Can you work these out from the model? Positions are in its coordinate system, mm. A direction names the side the tool comes from. Give positions to 0.01 mm unless a question says otherwise; leave off trailing zeros. Write each loop counter-clockwise with the first axis right and the second up, starting at its lowest first coordinate (ties: lowest second). Pieces come first, ordered by that corner, then holes.
```python
from build123d import *

# Parameters (mm, degrees)
BOSS_EXTRUDE1_DEPTH = 100
CUT_EXTRUDE1_DEPTH  = 100
BOSS_EXTRUDE2_DEPTH = 15
SKETCH4_W           = 40
SKETCH4_H           = 35
CUT_EXTRUDE2_DEPTH  = 137.950721064
SKETCH5_W           = 20
SKETCH5_H           = 15
BOSS_EXTRUDE3_DEPTH = 10
SKETCH6_W           = 20
SKETCH6_H           = 15
BOSS_EXTRUDE4_DEPTH = 10


with BuildPart() as part:
    # Sketch1 → Boss-Extrude1 (new body)
    with BuildSketch(Plane(origin=(0, 0, 0), x_dir=(1, 0, 0), z_dir=(0, 1, 0))):
        with BuildLine():
            Line((-10, 54.591666031), (-10, 39.591666031))
            Line((-10, 39.591666031), (-5, 39.591666031))
            Line((-5, 39.591666031), (-5, 24.591666031))
            Line((-5, 24.591666031), (-10, 24.591666031))
            Line((-10, 24.591666031), (-10, 0))
            ThreePointArc((-10, 0), (-7.071067812, -7.071067812), (0, -10))
            Line((0, -10), (20, -10))
            Line((20, -10), (20, -25))
            Line((20, -25), (-20, -25))
            Line((-20, -25), (-20, -51.771130952))
            ThreePointArc((-20, -51.771130952), (-55.256322222, 5.195079839), (-10, 54.591666031))
        make_face()
    extrude(amount=BOSS_EXTRUDE1_DEPTH)

    # Sketch2 → Cut-Extrude1 (cut)
    with BuildSketch(Plane(origin=(0, 0, 10), x_dir=(-1, 0, 0), z_dir=(0, 0, -1))):
        with BuildLine():
            Line((-5, 90.003555636), (-5, 10.003555636))
            ThreePointArc((-5, 10.003555636), (-10, 5.003555636), (-15, 10.003555636))
            Line((-15, 10.003555636), (-15, 90.003555636))
            ThreePointArc((-15, 90.003555636), (-10, 95.003555636), (-5, 90.003555636))
        make_face()
    extrude(amount=-CUT_EXTRUDE1_DEPTH, mode=Mode.SUBTRACT)

    # Sketch3 → Boss-Extrude2 (add)
    with BuildSketch(Plane(origin=(0, 100, 0), x_dir=(1, 0, 0), z_dir=(0, 1, 0))):
        with BuildLine():
            Line((20, -25), (20, -20))
            Line((20, -20), (-55.356937984, -3.982388364))
            ThreePointArc((-55.356937984, -3.982388364), (-44.616230288, -33.009725763), (-20, -51.771130952))
            Line((-20, -51.771130952), (-20, -25))
            Line((-20, -25), (20, -25))
        make_face()
    extrude(amount=BOSS_EXTRUDE2_DEPTH)

    # Sketch4 → Cut-Extrude2 (cut, through all)
    with BuildSketch(Plane(origin=(-5, 0, 0), x_dir=(0, 0, -1), z_dir=(1, 0, 0))):
        with Locations((34.591666031, 52.5)):
            Rectangle(SKETCH4_W, SKETCH4_H)
    extrude(amount=-CUT_EXTRUDE2_DEPTH, mode=Mode.SUBTRACT)

    # Sketch5 → Boss-Extrude3 (add)
    with BuildSketch(Plane(origin=(0, 100, 0), x_dir=(1, 0, 0), z_dir=(0, 1, 0))):
        with Locations((-15, 32.091666031)):
            Rectangle(SKETCH5_W, SKETCH5_H)
    extrude(amount=BOSS_EXTRUDE3_DEPTH)

    # Sketch6 → Boss-Extrude4 (add)
    with BuildSketch(Plane.XZ):
        with Locations((-15, -32.091666031)):
            Rectangle(SKETCH6_W, SKETCH6_H)
    extrude(amount=BOSS_EXTRUDE4_DEPTH)


solid = part.part
```
1) For faces 1 (the face through (0, 57, 25)), 2 (the face through (-8, 99, -24.592)), 3 (the face through (-24, 70, -30)), 4 (the face through (-5, 90, -32)), 5 (the face through (9.89, 5.005, 17.395)), which set-ups out of +Z, -Z, +X, -X, +Y, -Y let a thin tool reach every point of the face, with its end or its side?
Values follow:
face 1: +Z, +X, +Y, -Y
face 2: +X, +Y
face 3: -Z, +X, -X
face 4: -Z, +X, +Y, -Y
face 5: +Z, -Z
2) Suppose I cut it at C-C on x = 8. Write out the boundary of the cut face in (y, z).
Values follow:
outline: (0, 10) - (5.42, 10) - (5.42, 25) - (0, 25) - close; (94.59, 10) - (100, 10) - (100, 17.45) - (115, 17.45) - (115, 25) - (94.59, 25) - close
3) If we mould it in two halves opening along Z, with no side actions, what happens to faces 6 (the face through (-17.151, 107.395, 12.103)), 7 (the face through (-24, 35, -30)), 8 (the face through (-31, 52, -14.592)), 9 (the face through (-8, 3, -24.592))? For each: +Z half, -Z half, draft (parallel to the pull), parting line (faces both ways), or undercut.
Values follow:
face 6: undercut
face 7: draft
face 8: -Z half
face 9: undercut
4) Suppose I cut it at B-B on z = -45.5. Write out the boundary of the cut face in (x, y), plus the area to 3 significant figures.
Values follow:
outline: (-31.78, 0) - (-10, 0) - (-10, 35) - (-31.78, 35) - close; (-31.78, 70) - (-10, 70) - (-10, 100) - (-31.78, 100) - close
area: 1,420 mm2
5) Please list where these lines run through material, in increasing order: L1, parallel to Y at x = -23, z = -22.5; L2, parallel to Y at x = -19.5, z = -28; L3, parallel to X at y = 80.5, z = 22.
Values follow:
L1: y = 0 to 35, 70 to 100
L2: y = -10 to 35, 70 to 110
L3: x = -50.95 to 5, 15 to 20
6) For pin 1 Ø10 at (x, z) = (-29, -40.5) entering from +Y; pin 2 Ø2 at (y, z) = (30.5, 22.5) entering from -X; pin 3 Ø2 at (y, z) = (30.5, -8) entering from +X, each with a flat end and sliding along its axis, tell me the tip position at first contact or that it passes through.
Values follow:
pin 1: stops at y = 110
pin 2: stops at x = -51.17
pin 3: stops at x = -10
7) Suppose I cut it at A-A on y = 60.5. Write out the boundary of the cut face in (x, z), plus the area to 3 significant figures.
Values follow:
outline: (-53.55, -14.59) - (-10, -14.59) - (-10, 0) arc R10 cw to (0, 10) - (5, 10) - (5, 25) - (-20, 25) - (-20, 51.77) arc R55.5 ccw to start; (15, 10) - (20, 10) - (20, 25) - (15, 25) - close
area: 2,560 mm2
8) Suppose I cut it at D-D on y = 22. Write out the boundary of the cut face in (x, z).
Values follow:
outline: (-20, 25) - (-20, 51.77) arc R55.5 ccw to (-10, -54.59) - (-10, -39.59) - (-5, -39.59) - (-5, -24.59) - (-10, -24.59) - (-10, 0) arc R10 cw to (0, 10) - (5, 10) - (5, 25) - close; (15, 10) - (20, 10) - (20, 25) - (15, 25) - close
